Geometry check sheet. Reference: the model listing, model coordinates, mm. A direction names the side the tool comes from. Give positions to 0.01 mm unless a question says otherwise; leave off trailing zeros. Order: outer loops, then holes, each group sorted by start corner. A loop starts at its lowest first (then second) coordinate and runs counter-clockwise, first axis right, second up. Notation, with made-up numbers: M -13.5,31 L 19.5,31 A34 ccw 19.5,64 Z; hole C 24.25,39 d5. An arc over 180 degrees is marked long. Answer as CSV lines item,"result". Start each with the question number.
```python
from build123d import *

# Parameters (mm, degrees)
SKETCH_1_R          = 15
EXTRUDE_1_DEPTH     = 2
SKETCH_2_R          = 2
EXTRUDE_2_DEPTH     = 5
SKETCH_3_R          = 15
EXTRUDE_3_DEPTH     = 2
CUT_EXTRUDE_1_REACH = 11
SKETCH_4_R          = 1.5
SKETCH_4_R_2        = 2.8
SKETCH_5_R          = 2.8
CUT_EXTRUDE_2_DEPTH = 5


with BuildPart() as part:
    # 草图1 → 凸台-拉伸1 (new body)
    with BuildSketch(Plane.XY):
        Circle(SKETCH_1_R)
    extrude(amount=EXTRUDE_1_DEPTH)

    # 草图2 → 凸台-拉伸2 (add)
    with BuildSketch(Plane.XY.offset(2)):
        with Locations((11.655867717, 0)):
            Circle(SKETCH_2_R)
        with BuildLine():
            Line((8.655867717, 6.787927082), (8.655867717, -6.787927082))
            ThreePointArc((8.655867717, -6.787927082), (-11, 0), (8.655867717, 6.787927082))
        make_face()
    extrude(amount=EXTRUDE_2_DEPTH)

    # 草图3 → 凸台-拉伸3 (add)
    with BuildSketch(Plane.XY.offset(7)):
        Circle(SKETCH_3_R)
    extrude(amount=EXTRUDE_3_DEPTH)

    # 草图4 → 切除-拉伸1 (cut, up to next)
    with BuildSketch(Plane(origin=(0, 0, 0), x_dir=(-1, 0, 0), z_dir=(0, 0, -1)), mode=Mode.PRIVATE) as cut_extrude_1_sk1:
        with Locations((0, 7)):
            Circle(SKETCH_4_R)
    cut_extrude_1_tool1 = extrude(cut_extrude_1_sk1.sketch, amount=-CUT_EXTRUDE_1_REACH, mode=Mode.PRIVATE) & part.part
    add(cut_extrude_1_tool1.solids().sort_by_distance((0, 7, 0))[0], mode=Mode.SUBTRACT)
    # 草图4 → 切除-拉伸1 (cut, up to next)
    with BuildSketch(Plane(origin=(0, 0, 0), x_dir=(-1, 0, 0), z_dir=(0, 0, -1)), mode=Mode.PRIVATE) as cut_extrude_1_sk2:
        with Locations((0, -7)):
            Circle(SKETCH_4_R)
    cut_extrude_1_tool2 = extrude(cut_extrude_1_sk2.sketch, amount=-CUT_EXTRUDE_1_REACH, mode=Mode.PRIVATE) & part.part
    add(cut_extrude_1_tool2.solids().sort_by_distance((0, -7, 0))[0], mode=Mode.SUBTRACT)
    # 草图4 → 切除-拉伸1 (cut, up to next)
    with BuildSketch(Plane(origin=(0, 0, 0), x_dir=(-1, 0, 0), z_dir=(0, 0, -1)), mode=Mode.PRIVATE) as cut_extrude_1_sk3:
        with Locations((7, 0)):
            Circle(SKETCH_4_R)
    cut_extrude_1_tool3 = extrude(cut_extrude_1_sk3.sketch, amount=-CUT_EXTRUDE_1_REACH, mode=Mode.PRIVATE) & part.part
    add(cut_extrude_1_tool3.solids().sort_by_distance((-7, 0, 0))[0], mode=Mode.SUBTRACT)
    # 草图4 → 切除-拉伸1 (cut, up to next)
    with BuildSketch(Plane(origin=(0, 0, 0), x_dir=(-1, 0, 0), z_dir=(0, 0, -1)), mode=Mode.PRIVATE) as cut_extrude_1_sk4:
        with Locations((-7, 0)):
            Circle(SKETCH_4_R)
    cut_extrude_1_tool4 = extrude(cut_extrude_1_sk4.sketch, amount=-CUT_EXTRUDE_1_REACH, mode=Mode.PRIVATE) & part.part
    add(cut_extrude_1_tool4.solids().sort_by_distance((7, 0, 0))[0], mode=Mode.SUBTRACT)
    # 草图4 → 切除-拉伸1 (cut, up to next)
    with BuildSketch(Plane(origin=(0, 0, 0), x_dir=(-1, 0, 0), z_dir=(0, 0, -1)), mode=Mode.PRIVATE) as cut_extrude_1_sk5:
        Circle(SKETCH_4_R_2)
    cut_extrude_1_tool5 = extrude(cut_extrude_1_sk5.sketch, amount=-CUT_EXTRUDE_1_REACH, mode=Mode.PRIVATE) & part.part
    add(cut_extrude_1_tool5.solids().sort_by_distance((0, 0, 0))[0], mode=Mode.SUBTRACT)

    # 草图5 → 切除-拉伸2 (cut)
    with BuildSketch(Plane.XY.offset(9)):
        with Locations((0, 7)):
            Circle(SKETCH_5_R)
        with Locations((7, 0)):
            Circle(SKETCH_5_R)
        with Locations((-7, 0)):
            Circle(SKETCH_5_R)
        with Locations((0, -7)):
            Circle(SKETCH_5_R)
    extrude(amount=-CUT_EXTRUDE_2_DEPTH, mode=Mode.SUBTRACT)


solid = part.part
```
Item 1: Scan lines: line 1 along Y through (x, z) = (0, 1.75); line 2 along Y through (x, z) = (0, 7.75); line 3 along Z through (x, y) = (-10.25, -5.5). Record each from-to range of solid material in increasing order.
Item 2: Section check A-A on z = 3.25. Record the boundary of the cut face in (x, y).
Item 3: Section check D-D on z = 5.5. Record the boundary of the cut face in (x, y), then the cut area to 3 significant figures.
Item 4: Access from +Z, -Z, +X, -X, +Y, -Y to the whole of each face (thin tool, end or side, straight path). Record for faces 5 (the face through (8.5, 0.07, 1.97)), 6 (the face through (1.2, 5.8, 4)), 7 (the face through (13.564, 0.601, 4.465)).
Item 5: Depth check by flat-ended pin: pin 1 Ø1.5 at (y, z) = (-7.5, 6.5) entering from -X; pin 2 Ø4 at (y, z) = (3, 2.5) entering from -X; pin 3 Ø3.5 at (x, y) = (7, 1) entering from +Z; pin 4 Ø2.5 at (x, y) = (0, -7) entering from +Z. Enter the tip coordinate at first touch or a pass-through.
Item 6: Draft check along Z on faces 1 (the face through (5, 0, 4)), 2 (the face through (-0.607, -9.733, 6.535)), 3 (the face through (9, -3, 7)), 4 (the face through (3, 0, 0)). Enter one of: pulls with the +Z half, pulls with the -Z half, needs draft (parallel to the pull), parting line crosses it, or undercut.
Item 7: Section check B-B on y = -12. Record the boundary of the cut face in (x, z), then the cut area to 3 significant figures.
Item 8: Section check C-C on x = 0. Give the number of separate pieces and of enclosed holes in the cut face, then the cut area to 3 significant figures.
Numbers:
1,line 1,"-15 to -8.5, -5.5 to -2.8, 2.8 to 5.5, 8.5 to 15"
1,line 2,"-15 to -9.8, -4.2 to -2.8, 2.8 to 4.2, 9.8 to 15"
1,line 3,"0 to 2, 7 to 9"
2,outline,"M 8.66,-6.79 L 8.66,6.79 A11 ccw long Z; C 11.66,0 d4; hole C -7,0 d3; hole C 0,0 d5.6; hole C 0,-7 d3; hole C 0,7 d3; hole C 7,0 d3"
3,outline,"M 8.66,-6.79 L 8.66,-2.26 A2.8 cw long 8.66,2.26 L 8.66,6.79 A11 ccw long Z; M 9.74,-0.58 A2 ccw long 9.74,0.58 A2.8 cw Z; hole C -7,0 d5.6; hole C 0,-7 d5.6; hole C 0,0 d5.6; hole C 0,7 d5.6"
3,area,"251 mm2"
4,face 5,"+Z, -Z"
4,face 6,"+Z"
4,face 7,"none"
5,pin 1,"x = -13.3"
5,pin 2,"x = -14.96"
5,pin 3,"z = 4"
5,pin 4,"through"
6,face 1,"pulls with the +Z half"
6,face 2,"needs draft"
6,face 3,"undercut"
6,face 4,"pulls with the -Z half"
7,outline,"M -9,0 L 9,0 L 9,2 L -9,2 Z; M -9,7 L 9,7 L 9,9 L -9,9 Z"
7,area,"72.0 mm2"
8,separate pieces,"4"
8,enclosed holes,"0"
8,area,"99.6 mm2"
